Design review of the part built by this model. Coordinates are the model's own, in mm. A direction names the side the tool comes from. Coordinates: 2 decimals unless noted, no trailing zeros. Loops run counter-clockwise (first coordinate to the right, second up) from the corner with the lowest first, then second, coordinate; pieces in that order, holes last. Notation, with made-up numbers: (80, 43) -> (139, 43) arc R11 ccw to (139, 47) -> close; hole circle Ø11 at (80.25, 53). An arc over 180 degrees is marked (long way). Use one line per item in the form item = value. Start each with the question number.
1. Consider section A-A (x = 20). State the section outline as (y, z) points.
2. Consider section B-B (z = 2.25). State the section outline as (x, y) points.
3. Wall thickness on line 1 (Y direction, x = 10.5, z = 5.5); line 2 (X direction, y = 16, z = 4); line 3 (Z direction, x = -20, y = 5.5): over which ranges is each line inside the solid? List them lowest first. Write a range as from..to.
4. Consider section D-D (x = -3.5). State the section outline as (y, z) points.
5. For pin 1 (1.5 mm diameter, centred on x = -14, y = 16.5, fed in from +Z); pin 2 (5 mm diameter, centred on y = 4.5, z = 6, fed in from +X); pin 3 (3 mm diameter, centred on x = 4, z = 7, fed in from +Y), all flat-tipped, find the tip position at first contact; note any pin that passes through.
6. The part is to be moulded in two halves that separate along Z. For faces 3 (the face through (15.85, 6.26, -2.83)), 4 (the face through (0, 6, -13.623)), 5 (the face through (-16.7, 25.4, 2.1)), say which applies: released by +Z, released by -Z, zero draft, split by the parting line, or undercut.
7. Consider section C-C (y = 11). State the section outline as (x, z) points.
8. Machinability: for faces 1 (the face through (-34.274, 15.344, 3.942)), 2 (the face through (34.604, 6.261, -1.202)), which of the approach directions +Z, -Z, +X, -X, +Y, -Y give a long, thin tool a straight path to every point of the face, cutting with its end or side? Answer none if there is none.
Autodesk Inventor part; units mm, degrees
ref_plane "YZ Plane" through (0, 0, 0) normal (1, 0, 0) x (0, 1, 0)
ref_plane "XZ Plane" through (0, 0, 0) normal (0, 1, 0) x (-1, 0, 0)
ref_plane "XY Plane" through (0, 0, 0) normal (0, 0, 1) x (1, 0, 0)
sketch "Sketch1" plane through (0, 0, 0) normal (0, 1, 0) x (-1, 0, 0)
  line L0 (22.5427, 11.7774) -> (-21.9073, 11.7774)
  line L1 (-21.9073, 11.7774) -> (-21.9073, -13.6226)
  line L2 (-21.9073, -13.6226) -> (22.5427, -13.6226)
  line L3 (22.5427, -13.6226) -> (22.5427, 11.7774)
  circle A0 centre (-21.9073, -0.9226) radius 12.7
  circle A1 centre (-21.9073, -0.9226) radius 6.35
  circle A2 centre (22.5427, -0.9226) radius 12.7
  circle A3 centre (22.5427, -0.9226) radius 6.35
  point P0 (0, 0)
  dimension "d0" = 44.45
  dimension "d1" = 25.4
  dimension "d5" = 12.7
  dimension "d8" = 25.4
  dimension "d9" = 12.7
extrude "Extrusion2" add sketch "Sketch1" along normal blind 12.7 contours A2 L2 A0 L0 | L3 A3 A2 | A0 L1 A1 | L3 A3 | A1 L1 picked at (21.023, -11.3214) picked at (-14.3032, 6.3463) picked at (19.6489, 0.8427) picked at (-19.8437, -0.4516)
extrude "Extrusion3" add sketch "Sketch1" along normal blind 12.7 contours A0 L1 A1 | L1 A1 A0
extrude "Extrusion4" cut sketch "Sketch1" along normal blind 12.7 contours A1 L1 | L1 A1
extrude "Extrusion5" add sketch "Sketch1" along normal blind 25.4 contours A2 L3 A3 | L3 A3 A2
extrude "Extrusion6" cut sketch "Sketch1" against normal blind 25.4 contours A3 L3 | L3 A3
extrude "Extrusion7" cut sketch "Sketch1" along normal blind 25.4 contours A3 L3 | L3 A3
Geometry check:
q1.outline = (0, -13.62) -> (12.7, -13.62) -> (12.7, -6.98) -> (0, -6.98) -> close; (0, 5.13) -> (12.7, 5.13) -> (12.7, 11.78) -> (0, 11.78) -> close
q2.outline = (-34.84, 0) -> (-28.04, 0) -> (-28.04, 25.4) -> (-34.84, 25.4) -> close; (-17.04, 0) -> (16.41, 0) -> (16.41, 12.7) -> (-10.25, 12.7) -> (-10.25, 25.4) -> (-17.04, 25.4) -> close; (27.41, 0) -> (34.2, 0) -> (34.2, 12.7) -> (27.41, 12.7) -> close
q3.line_1 = 0..12.7
q3.line_2 = -34.25..-26.55, -18.53..-10.84
q3.line_3 = -13.62..-6.74, 4.9..11.78
q4.outline = (0, -13.62) -> (12.7, -13.62) -> (12.7, 11.78) -> (0, 11.78) -> close
q5.pin_1 = 9.11
q5.pin_2 = 33.81
q5.pin_3 = 12.7
q6.face_3 = undercut
q6.face_4 = released by -Z
q6.face_5 = zero draft
q7.outline = (-22.54, -13.62) -> (21.91, -13.62) arc R12.7 ccw to (21.91, 11.78) -> (-22.54, 11.78) arc R12.7 ccw to start; hole circle Ø12.7 at (-22.54, -0.92); hole circle Ø12.7 at (21.91, -0.92)
q8.face_1 = +Y
q8.face_2 = +X, +Y, -Y
